Check sheet for the drawn part. Datum: minimum x, y, z corner. Units: mm. Round coordinates to 2 decimals unless told otherwise and drop trailing zeros. Write each loop counter-clockwise with the first axis right and the second up, starting at its lowest first coordinate (ties: lowest second). Pieces come first, ordered by that corner, then holes. Notation, with made-up numbers: (45, 44.5) - (97, 44.5) arc R7 ccw to (97, 48.5) - close; hole circle Ø9 at (4, -31). An arc over 180 degrees is marked (long way). Answer as a JSON object with one key per item and string values.
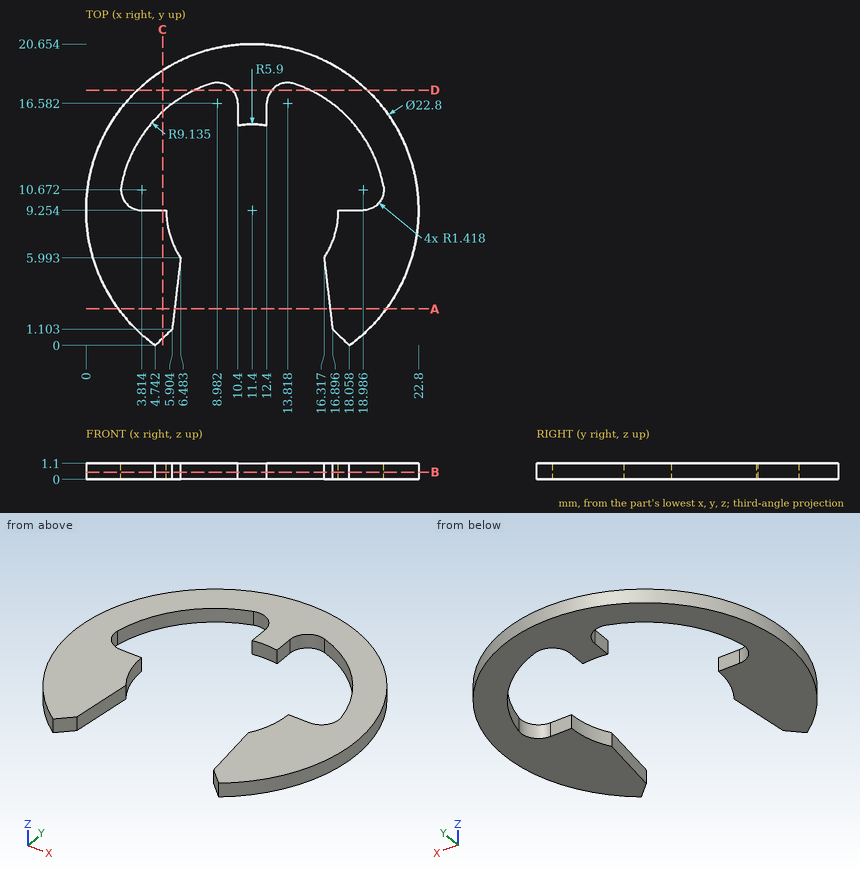
1. Cross-section at B-B (z = 0.5). Record the boundary of the cut face in (x, y) (1 decimal).
Completed:
{"outline": "(2.4, 10.9) arc R9.1 cw to (8.5, 17.9) arc R1.4 cw to (10.4, 16.6) - (10.4, 15.1) arc R5.9 cw to (12.4, 15.1) - (12.4, 16.6) arc R1.4 cw to (14.3, 17.9) arc R9.1 cw to (20.4, 10.9) arc R1.4 cw to (19, 9.3) - (17.3, 9.3) arc R5.9 cw to (16.3, 6) - (16.9, 1.1) - (18.1, 0) arc R11.4 ccw (long way) to (4.7, 0) - (5.9, 1.1) - (6.5, 6) arc R5.9 cw to (5.5, 9.3) - (3.8, 9.3) arc R1.4 cw to start"}
2. Cross-section at C-C (x = 5.25). Record the boundary of the cut face in (y, z) (1 decimal).
Completed:
{"outline": "(0.5, 0) - (9.3, 0) - (9.3, 1.1) - (0.5, 1.1) - close; (16, 0) - (18.9, 0) - (18.9, 1.1) - (16, 1.1) - close"}
3. Go/stop test with flat-tipped pins: pin 1 (0.6 mm diameter, centred on y = 16, z = 0.5, fed in from -X); pin 2 (0.6 mm diameter, centred on y = 15.5, z = 0.5, fed in from +X). Record where each tip stops, or that it passes through.
Completed:
{"pin 1": "stops at x = 2", "pin 2": "stops at x = 21.13"}
4. Cross-section at D-D (y = 17.5). Record the boundary of the cut face in (x, z), plus the area to 3 significant figures.
Completed:
{"outline": "(3.53, 0) - (7.47, 0) - (7.47, 1.1) - (3.53, 1.1) - close; (10.06, 0) - (12.74, 0) - (12.74, 1.1) - (10.06, 1.1) - close; (15.33, 0) - (19.27, 0) - (19.27, 1.1) - (15.33, 1.1) - close", "area": "11.6 mm^2"}
5. Cross-section at A-A (y = 2.5). Record the boundary of the cut face in (x, z).
Completed:
{"outline": "(2.22, 0) - (6.07, 0) - (6.07, 1.1) - (2.22, 1.1) - close; (16.73, 0) - (20.58, 0) - (20.58, 1.1) - (16.73, 1.1) - close"}
6. Material ranges on probe 1 along X at (y, z) = (17.25, 0.8) (1 decimal); probe 2 along X at (y, z) = (16.25, 0.2) (1 decimal); probe 3 along X at (y, z) = (8.25, 0.6) (1 decimal), recorded low to high. Write a range as from..to.
Completed:
{"probe 1": "x = 3.3..7, 10.2..12.6, 15.8..19.5", "probe 2": "x = 2.4..5.5, 10.4..12.4, 17.3..20.4", "probe 3": "x = 0..5.6, 17.2..22.8"}
